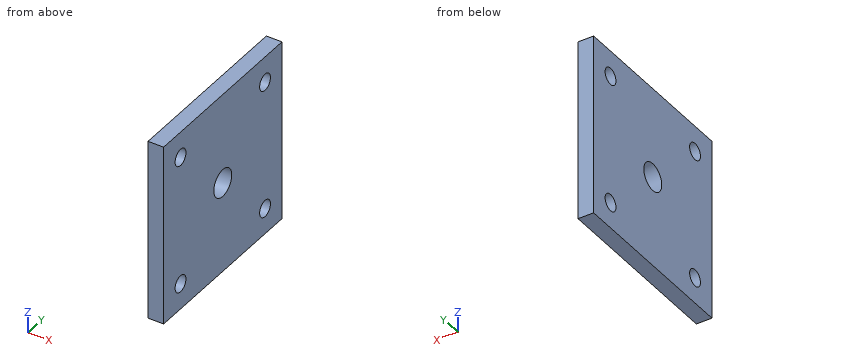
```python
from build123d import *

# Parameters (mm, degrees)
SKETCH1_W           = 35
SKETCH1_H           = 35
BOSS_EXTRUDE1_DEPTH = 3
SKETCH2_R           = 1.6
CUT_EXTRUDE1_DEPTH  = 25.929901725
SKETCH3_R           = 2.65
CUT_EXTRUDE2_DEPTH  = 25.929901725


with BuildPart() as part:
    # Sketch1 → Boss-Extrude1 (new body)
    with BuildSketch(Plane(origin=(0, 0, 0), x_dir=(0, 0, -1), z_dir=(1, 0, 0))):
        Rectangle(SKETCH1_W, SKETCH1_H)
    extrude(amount=BOSS_EXTRUDE1_DEPTH)

    # Sketch2 → Cut-Extrude1 (cut, through all)
    with BuildSketch(Plane.ZY):
        with Locations((-12.5, 12.5)):
            Circle(SKETCH2_R)
        with Locations((-12.5, -12.5)):
            Circle(SKETCH2_R)
        with Locations((12.5, -12.5)):
            Circle(SKETCH2_R)
        with Locations((12.5, 12.5)):
            Circle(SKETCH2_R)
    extrude(amount=-CUT_EXTRUDE1_DEPTH, mode=Mode.SUBTRACT)

    # Sketch3 → Cut-Extrude2 (cut, through all)
    with BuildSketch(Plane.ZY):
        Circle(SKETCH3_R)
    extrude(amount=-CUT_EXTRUDE2_DEPTH, mode=Mode.SUBTRACT)


solid = part.part
```
Check sheet for the modelled part. Datum: model origin and axes. Units: mm. Round coordinates to 2 decimals unless told otherwise and drop trailing zeros. Order: outer loops, then holes, each group sorted by start corner. A loop starts at its lowest first (then second) coordinate and runs counter-clockwise, first axis right, second up. Notation, with made-up numbers: (27.25, 44.25) - (53.25, 44.25) arc R23 ccw to (53.25, 63.25) - close; hole circle Ø4 at (-20, 22.5). An arc over 180 degrees is marked (long way). Write item = value, one per line.
Q1. Thickness scan on line 1 along Y through (x, z) = (1.9, 12.5); line 2 along Z through (x, y) = (1.15, -11.5); line 3 along Z through (x, y) = (0.6, -13). Record the ranges inside material, lowest first.
Computed:
line_1 = -17.5 to -14.1, -10.9 to 10.9, 14.1 to 17.5
line_2 = -17.5 to -13.75, -11.25 to 11.25, 13.75 to 17.5
line_3 = -17.5 to -14.02, -10.98 to 10.98, 14.02 to 17.5
Q2. Section check D-D (y = 1.5). Record the boundary of the cut face in (x, z), and give its area (3 significant figures).
Computed:
outline = (0, -17.5) - (3, -17.5) - (3, -2.18) - (0, -2.18) - close; (0, 2.18) - (3, 2.18) - (3, 17.5) - (0, 17.5) - close
area = 91.9 mm^2
Q3. Go/stop test with a flat-tipped pin: pin 1 (3 mm diameter, centred on y = 0, z = 0, fed in from -X). Record where the tip stops, or that it passes through.
Computed:
pin_1 = through
Q4. Section check B-B (z = 0). Record the boundary of the cut face in (x, y).
Computed:
outline = (0, -17.5) - (3, -17.5) - (3, -2.65) - (0, -2.65) - close; (0, 2.65) - (3, 2.65) - (3, 17.5) - (0, 17.5) - close
Q5. Section check A-A (z = 12.5). Record the boundary of the cut face in (x, y), and give its area (3 significant figures).
Computed:
outline = (0, -17.5) - (3, -17.5) - (3, -14.1) - (0, -14.1) - close; (0, -10.9) - (3, -10.9) - (3, 10.9) - (0, 10.9) - close; (0, 14.1) - (3, 14.1) - (3, 17.5) - (0, 17.5) - close
area = 85.8 mm^2
